```python
from build123d import *

# Parameters (mm, degrees)
SKETCH1_W               = 80
SKETCH1_H               = 42
BOSS_EXTRUDE1_DEPTH     = 25
SKETCH6_W               = 78
SKETCH6_H               = 40
CUT_EXTRUDE6_DEPTH      = 24
CUT_EXTRUDE7_REACH      = 53.157
SKETCH7_W               = 33.5
SKETCH7_H               = 20
SKETCH8_W               = 5
SKETCH8_H               = 6
BOSS_EXTRUDE2_DEPTH     = 4
SKETCH9_W               = 9.5
SKETCH9_H               = 25.25
BOSS_EXTRUDE3_DEPTH     = 1
FILLET1_R               = 1
FILLET3_R               = 2
CUT_EXTRUDE8_REACH      = 87.481
SKETCH18_W              = 20
SKETCH18_H              = 2.25
SKETCH18_H_2            = 3
BOSS_EXTRUDE5_DEPTH     = 5.5
FILLET5_R               = 2
CUT_EXTRUDE12_REACH     = 88.406
BOSS_EXTRUDE6_DEPTH     = 6
CUT_EXTRUDE13_REACH     = 53.633
SKETCH22_R              = 1.75
MIRROR3_COPY_1_DEPTH    = 6
MIRROR3_COPY_2_REACH    = 53.633
MIRROR3_COPY_2_SKETCH_R = 1.75
FILLET6_R               = 2
BOSS_EXTRUDE7_DEPTH     = 1
CUT_EXTRUDE14_REACH     = 88.406
SKETCH24_W              = 20
SKETCH24_H              = 13


with BuildPart() as part:
    # Sketch1 → Boss-Extrude1 (new body)
    with BuildSketch(Plane(origin=(0, 0, 0), x_dir=(1, 0, 0), z_dir=(0, 1, 0))):
        Rectangle(SKETCH1_W, SKETCH1_H)
    extrude(amount=BOSS_EXTRUDE1_DEPTH)

    # Sketch6 → Cut-Extrude6 (cut)
    with BuildSketch(Plane(origin=(0, 25, 0), x_dir=(1, 0, 0), z_dir=(0, 1, 0))):
        Rectangle(SKETCH6_W, SKETCH6_H)
    extrude(amount=-CUT_EXTRUDE6_DEPTH, mode=Mode.SUBTRACT)

    # Sketch7 → Cut-Extrude7 (cut, up to next)
    with BuildSketch(Plane(origin=(0, 1, 0), x_dir=(1, 0, 0), z_dir=(0, 1, 0)), mode=Mode.PRIVATE) as cut_extrude7_sk1:
        with Locations((-7.75, 7.75)):
            Rectangle(SKETCH7_W, SKETCH7_H)
    cut_extrude7_tool1 = extrude(cut_extrude7_sk1.sketch, amount=-CUT_EXTRUDE7_REACH, mode=Mode.PRIVATE) & part.part
    add(cut_extrude7_tool1.solids().sort_by_distance((-7.75, 1, -7.75))[0], mode=Mode.SUBTRACT)

    # Sketch8 → Boss-Extrude2 (add)
    with BuildSketch(Plane(origin=(0, 1, 0), x_dir=(1, 0, 0), z_dir=(0, 1, 0))):
        with Locations((-27, 7.75)):
            Rectangle(SKETCH8_W, SKETCH8_H)
    extrude(amount=BOSS_EXTRUDE2_DEPTH)

    # Sketch9 → Boss-Extrude3 (add)
    with BuildSketch(Plane(origin=(0, 1, 0), x_dir=(1, 0, 0), z_dir=(0, 1, 0))):
        with Locations((-34.25, 7.375)):
            Rectangle(SKETCH9_W, SKETCH9_H)
    extrude(amount=BOSS_EXTRUDE3_DEPTH)

    # Fillet1
    fillet1_edges = [part.edges().sort_by_distance(p)[0] for p in [
        (-27, 1, -10.75),
        (-27, 1, -4.75),
    ]]
    fillet(fillet1_edges, radius=FILLET1_R)

    # Fillet3
    fillet3_edges = [part.edges().sort_by_distance(p)[0] for p in [
        (-39, 13, 20),
        (39, 13, 20),
        (39, 13, -20),
        (-39, 13.5, -20),
        (40, 12.5, 21),
        (-40, 12.5, 21),
        (-40, 12.5, -21),
        (40, 12.5, -21),
    ]]
    fillet(fillet3_edges, radius=FILLET3_R)

    # Sketch12 → Cut-Extrude8 (cut, up to next)
    with BuildSketch(Plane(origin=(-39, 0, 0), x_dir=(0, 0, -1), z_dir=(1, 0, 0)), mode=Mode.PRIVATE) as cut_extrude8_sk1:
        with BuildLine():
            Line((5, 6.5), (10.5, 6.5))
            ThreePointArc((10.5, 6.5), (12.5, 4.5), (10.5, 2.5))
            Line((10.5, 2.5), (5, 2.5))
            ThreePointArc((5, 2.5), (3, 4.5), (5, 6.5))
        make_face()
    cut_extrude8_tool1 = extrude(cut_extrude8_sk1.sketch, amount=-CUT_EXTRUDE8_REACH, mode=Mode.PRIVATE) & part.part
    add(cut_extrude8_tool1.solids().sort_by_distance((-39, 4.5, -7.75))[0], mode=Mode.SUBTRACT)

    # Sketch18 → Boss-Extrude5 (add)
    with BuildSketch(Plane(origin=(0, 1, 0), x_dir=(1, 0, 0), z_dir=(0, 1, 0))):
        with Locations((-1, 18.875)):
            Rectangle(SKETCH18_W, SKETCH18_H)
        with Locations((-1, -3.75)):
            Rectangle(SKETCH18_W, SKETCH18_H_2)
    extrude(amount=BOSS_EXTRUDE5_DEPTH)

    # Fillet5
    fillet5_edges = [part.edges().sort_by_distance(p)[0] for p in [
        (9, 1, -18.875),
        (-11, 1, -18.875),
        (9, 6.5, -18.875),
        (-11, 6.5, -18.875),
        (9, 1, 3.75),
        (-11, 1, 3.75),
        (9, 6.5, 3.75),
        (-11, 6.5, 3.75),
    ]]
    fillet(fillet5_edges, radius=FILLET5_R)

    # Sketch19 → Cut-Extrude12 (cut, up to next)
    with BuildSketch(Plane.ZY.offset(40), mode=Mode.PRIVATE) as cut_extrude12_sk1:
        with BuildLine():
            Line((10, 8.75), (10, 6.25))
            ThreePointArc((10, 6.25), (16.25, 7.5), (10, 8.75))
        make_face()
    cut_extrude12_tool1 = extrude(cut_extrude12_sk1.sketch, amount=-CUT_EXTRUDE12_REACH, mode=Mode.PRIVATE) & part.part
    add(cut_extrude12_tool1.solids().sort_by_distance((-40, 7.5, 13.039742))[0], mode=Mode.SUBTRACT)

    # Sketch20 → Boss-Extrude6 (add)
    with BuildSketch(Plane(origin=(0, 25, 0), x_dir=(1, 0, 0), z_dir=(0, 1, 0))):
        with BuildLine():
            Line((-34.5, 20), (-37, 20))
            ThreePointArc((-37, 20), (-38.414213562, 19.414213562), (-39, 18))
            Line((-39, 18), (-39, 15.5))
            Line((-39, 15.5), (-37, 15.5))
            ThreePointArc((-37, 15.5), (-35.232233047, 16.232233047), (-34.5, 18))
            Line((-34.5, 18), (-34.5, 20))
        make_face()
    boss_extrude6 = extrude(amount=-BOSS_EXTRUDE6_DEPTH)

    # Sketch22 → Cut-Extrude13 (cut, up to next)
    with BuildSketch(Plane(origin=(0, 25, 0), x_dir=(1, 0, 0), z_dir=(0, 1, 0)), mode=Mode.PRIVATE) as cut_extrude13_sk1:
        with Locations(Location((-37, 18, 0), (0, 0, 270))):
            Circle(SKETCH22_R)
    cut_extrude13_tool1 = extrude(cut_extrude13_sk1.sketch, amount=-CUT_EXTRUDE13_REACH, mode=Mode.PRIVATE) & part.part
    cut_extrude13 = cut_extrude13_tool1.solids().sort_by_distance((-37, 25, -18))[0]
    add(cut_extrude13, mode=Mode.SUBTRACT)

    # Mirror1: Boss-Extrude6, Cut-Extrude13 across plane
    add(boss_extrude6.mirror(Plane.XY))
    add(cut_extrude13.mirror(Plane.XY), mode=Mode.SUBTRACT)

    # Mirror3: Boss-Extrude6, Cut-Extrude13 across plane
    add(boss_extrude6.mirror(Plane(origin=(0, 0, 0), x_dir=(0, 0, 1), z_dir=(1, 0, 0))))
    add(cut_extrude13.mirror(Plane(origin=(0, 0, 0), x_dir=(0, 0, 1), z_dir=(1, 0, 0))), mode=Mode.SUBTRACT)

    # Mirror3 copy 1 sketch → Mirror3 copy 1 (add)
    with BuildSketch(Plane(origin=(0, 25, 0), x_dir=(-1, 0, 0), z_dir=(0, 1, 0))):
        with BuildLine():
            Line((-34.5, 20), (-37, 20))
            ThreePointArc((-37, 20), (-38.414213562, 19.414213562), (-39, 18))
            Line((-39, 18), (-39, 15.5))
            Line((-39, 15.5), (-37, 15.5))
            ThreePointArc((-37, 15.5), (-35.232233047, 16.232233047), (-34.5, 18))
            Line((-34.5, 18), (-34.5, 20))
        make_face()
    extrude(amount=-MIRROR3_COPY_1_DEPTH)

    # Mirror3 copy 2 sketch → Mirror3 copy 2 (cut, up to next)
    with BuildSketch(Plane(origin=(0, 25, 0), x_dir=(-1, 0, 0), z_dir=(0, 1, 0)), mode=Mode.PRIVATE) as mirror3_copy_2_sk1:
        with Locations(Location((-37, 18, 0), (0, 0, 270))):
            Circle(MIRROR3_COPY_2_SKETCH_R)
    mirror3_copy_2_tool1 = extrude(mirror3_copy_2_sk1.sketch, amount=-MIRROR3_COPY_2_REACH, mode=Mode.PRIVATE) & part.part
    add(mirror3_copy_2_tool1.solids().sort_by_distance((37, 25, 18))[0], mode=Mode.SUBTRACT)

    # Fillet6
    fillet6_edges = [part.edges().sort_by_distance(p)[0] for p in [
        (0, 0, -21),
        (40, 0, 0),
        (0, 0, 21),
        (-40, 0, 0),
        (39.414213562, 0, 20.414213562),
        (-39.414213562, 0, 20.414213562),
        (-39.414213562, 0, -20.414213562),
        (39.414213562, 0, -20.414213562),
    ]]
    fillet(fillet6_edges, radius=FILLET6_R)

    # Sketch23 → Boss-Extrude7 (add)
    with BuildSketch(Plane.XZ):
        Polygon((-20.5, 2.25), (-20.5, -13.25), (6.5, -13.25), (6.5, 2.25), (9, 2.25), (9, -17.75), (-24.5, -17.75), (-24.5, 2.25), align=None)
    extrude(amount=-BOSS_EXTRUDE7_DEPTH)

    # Sketch24 → Cut-Extrude14 (cut, up to next)
    with BuildSketch(Plane(origin=(40, 0, 0), x_dir=(0, 0, -1), z_dir=(1, 0, 0)), mode=Mode.PRIVATE) as cut_extrude14_sk1:
        with Locations((-8, 10.5)):
            Rectangle(SKETCH24_W, SKETCH24_H)
    cut_extrude14_tool1 = extrude(cut_extrude14_sk1.sketch, amount=-CUT_EXTRUDE14_REACH, mode=Mode.PRIVATE) & part.part
    add(cut_extrude14_tool1.solids().sort_by_distance((40, 10.5, 8))[0], mode=Mode.SUBTRACT)


solid = part.part
```
Read the model definition and answer for the solid it produces. Units are mm, in the model's axes. A direction names the side the tool comes from. Give positions to 0.01 mm unless a question says otherwise; leave off trailing zeros. Order: outer loops, then holes, each group sorted by start corner. A loop starts at its lowest first (then second) coordinate and runs counter-clockwise, first axis right, second up. Notation, with made-up numbers: (21, 61) -> (66, 61) arc R24 ccw to (66, 97) -> close; hole circle Ø2 at (89, 10). An arc over 180 degrees is marked (long way). One line per item, written item: value. Start each with the question number.
(1) The part is cut by section D-D (y = 22.5). Determine the outline of the cut face in (x, z), and give its area (3 significant figures).
(2) The part is cut by section A-A (z = -6.5). Determine the outline of the cut face in (x, y).
(3) A tool of negligible diameter and unlimited length cuts with its end or side. For faces 1 (the cylindrical face through (8.43, 5.9, 3.73)), 2 (the cylindrical face through (-38.43, 10.38, -19.4)), 3 (the cylindrical face through (-38.71, 22.04, 18.38)), from which of +Z, -Z, +X, -X, +Y, -Y can it reach the whole face along a straight path? Write none if from no direction.
(4) Straight lines are drawn through the part: L1, parallel to X at y = 21, z = 18; L2, parallel to Z at x = -14.5, y = 3; L3, parallel to X at y = 20.75, z = 19. For each, find the intervals that lie inside material, in ascending order.
(5) For a pull along Z with two mould halves and no side action, classify faces 4 (the flat face through (38, 22, 15.5)), 5 (the cylindrical face through (39.4, 13.66, 20.43)), 6 (the cylindrical face through (-11.6, 1.57, 3.73)), 7 (the flat face through (0.2, 25, 20.3)) as released by +Z, released by -Z, zero draft, split by the parting line, or undercut.
(6) The part is cut by section B-B (y = 7.5). Determine the outline of the cut face in (x, z).
(7) Flat-ended cylindrical pins translate along their axes: P1, Ø8, axis at x = -8.5, z = 13, coming from the +Y side; P2, Ø5, axis at y = 11, z = 11.5, coming from the +X side; P3, Ø2.5, axis at x = -26, z = -8.5, coming from the +Y side. Find the tip coordinate at first contact, or state that the pin passes through.
(8) The part is cut by section C-C (z = 3.5). Determine the outline of the cut face in (x, y).
Taken from the geometry:
1. outline: (-40, -19) arc R2 ccw to (-38, -21) -> (38, -21) arc R2 ccw to (40, -19) -> (40, 19) arc R2 ccw to (38, 21) -> (-38, 21) arc R2 ccw to (-40, 19) -> close; hole (-39, -15.5) -> (-37, -15.5) arc R2.5 cw to (-34.5, -18) -> (-34.5, -20) -> (34.5, -20) -> (34.5, -18) arc R2.5 cw to (37, -15.5) -> (39, -15.5) -> (39, 15.5) -> (37, 15.5) arc R2.5 cw to (34.5, 18) -> (34.5, 20) -> (-34.5, 20) -> (-34.5, 18) arc R2.5 cw to (-37, 15.5) -> (-39, 15.5) -> close; hole circle Ø3.5 at (-37, -18); hole circle Ø3.5 at (-37, 18); hole circle Ø3.5 at (37, -18); hole circle Ø3.5 at (37, 18)
1. area: 274 mm^2
2. outline: (-40, 2) arc R2 ccw to (-38, 0) -> (-20.5, 0) -> (-20.5, 1) -> (-24.5, 1) -> (-24.5, 5) -> (-29.5, 5) -> (-29.5, 2) -> (-39, 2) -> (-39, 2.5) -> (-40, 2.5) -> close; (-40, 6.5) -> (-39, 6.5) -> (-39, 25) -> (-40, 25) -> close; (6.5, 0) -> (38, 0) arc R2 ccw to (40, 2) -> (40, 25) -> (39, 25) -> (39, 1) -> (6.5, 1) -> close
3. face 1: +X, +Y
3. face 2: none
3. face 3: +Y
4. L1: -40 to -38.75, -35.25 to -34.5, 34.5 to 35.25, 38.75 to 40
4. L2: -21 to -20, 20 to 21
4. L3: -40 to -38.44, -35.56 to -34.5, 34.5 to 35.56, 38.44 to 40
5. face 4: undercut
5. face 5: released by +Z
5. face 6: undercut
5. face 7: zero draft
6. outline: (-40, -19) arc R2 ccw to (-38, -21) -> (38, -21) arc R2 ccw to (40, -19) -> (40, -2) -> (39, -2) -> (39, -18) arc R2 cw to (37, -20) -> (-37, -20) arc R2 cw to (-39, -18) -> (-39, 10) -> (-40, 10) -> close; (-40, 16.25) -> (-39, 16.25) -> (-39, 18) arc R2 cw to (-37, 20) -> (37, 20) arc R2 cw to (39, 18) -> (40, 18) -> (40, 19) arc R2 ccw to (38, 21) -> (-38, 21) arc R2 ccw to (-40, 19) -> close
7. P1: y = 1
7. P2: x = -39
7. P3: y = 5
8. outline: (-40, 2) arc R2 ccw to (-38, 0) -> (38, 0) arc R2 ccw to (40, 2) -> (40, 4) -> (39, 4) -> (39, 1) -> (11, 1) arc R2 cw to (9, 3) -> (9, 4.5) arc R2 ccw to (7, 6.5) -> (-9, 6.5) arc R2 ccw to (-11, 4.5) -> (-11, 3) arc R2 cw to (-13, 1) -> (-29.5, 1) -> (-29.5, 2) -> (-39, 2) -> (-39, 25) -> (-40, 25) -> close; (39, 17) -> (40, 17) -> (40, 25) -> (39, 25) -> close
